Geometry: final body of the model. Coordinates: model frame, mm. Face numbers are marked on the shaded views. A direction names the side the tool comes from. Give positions to 0.01 mm unless a question says otherwise; leave off trailing zeros. Loops run counter-clockwise (first coordinate to the right, second up) from the corner with the lowest first, then second, coordinate; pieces in that order, holes last. Notation, with made-up numbers: (3.5, -23.5) - (16.5, -23.5) arc R27 cw to (16.5, 12.5) - close; hole circle Ø3 at (55, 82.5). An arc over 180 degrees is marked (long way). Use CSV: the item, a comma, the result in double quotes. Start each with the question number.
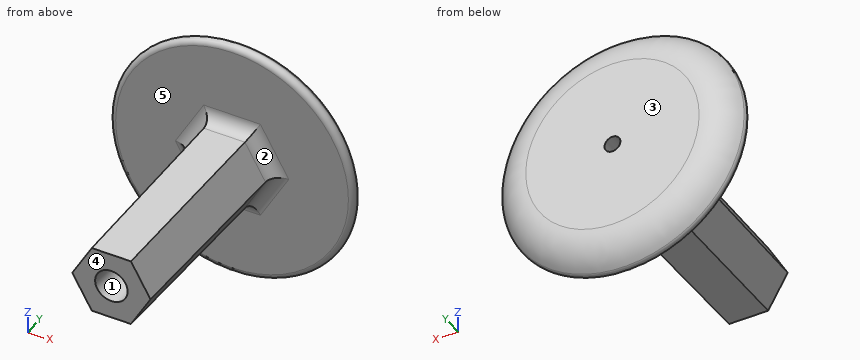
```python
from build123d import *

# Parameters (mm, degrees)
SHAFT_DEPTH          = 22.352
DRAFT_ON_SHAFT_ANGLE = 0.5
SKETCH3_R            = 1.524
THRU_HOLE_DEPTH      = 28.574862156
THRU_HOLE_DRAFT      = -2
FILLET1_R            = 1.27


with BuildPart() as part:
    # Sketch1 → Head (revolve)
    with BuildSketch(Plane.XY, mode=Mode.PRIVATE) as head_sk:
        with BuildLine():
            Line((0, 0), (10.910430592, 0))
            ThreePointArc((10.910430592, 0), (11.355976066, 0.263964694), (11.338496837, 0.781538462))
            ThreePointArc((11.338496837, 0.781538462), (9.958264798, 2.071591054), (8.128, 2.54))
            Line((8.128, 2.54), (0, 2.54))
            Line((0, 2.54), (0, 0))
        make_face()
    revolve(head_sk.sketch.rotate(Axis((0, 2.54, 0), (0, -1, 0)), 180), axis=Axis((0, 2.54, 0), (0, -1, 0)))

    # Sketch2 → Shaft (add)
    with BuildSketch(Plane(origin=(0, 2.54, 0), x_dir=(-1, 0, 0), z_dir=(0, 1, 0))):
        Polygon((1.833087105, -3.175), (-1.833087105, -3.175), (-3.666174209, 0), (-1.833087105, 3.175), (1.833087105, 3.175), (3.666174209, 0), align=None)
    extrude(amount=-SHAFT_DEPTH)

    # Draft on Shaft
    draft_on_shaft_faces = [part.faces().sort_by_distance(p)[0] for p in [
        (0, -9.906, 3.175),
        (2.749630657, -9.906, 1.5875),
        (2.749630657, -9.906, -1.5875),
        (0, -9.906, -3.175),
        (-2.749630657, -9.906, -1.5875),
        (-2.749630657, -9.906, 1.5875),
    ]]
    draft(draft_on_shaft_faces, Plane(origin=(5.499261314, -19.812, 3.175), x_dir=(-1, 0, 0), z_dir=(0, -1, 0)), DRAFT_ON_SHAFT_ANGLE)


with BuildPart() as thru_hole_tool:
    # Sketch3 → Thru Hole (with draft: the straight prism first)
    with BuildSketch(Plane.XZ.offset(19.812)):
        Circle(SKETCH3_R)
    extrude(amount=-THRU_HOLE_DEPTH)
    # Thru Hole: the draft: its side faces are tilted about the plane it starts from
    thru_hole_sides = [thru_hole_tool.faces().sort_by_distance(p)[0] for p in [
        (-1.524, -5.524568922, 0),
    ]]
    draft(thru_hole_sides, Plane.XZ.offset(19.812), THRU_HOLE_DRAFT)


with BuildPart() as part_1:
    add(part.part)

    # Thru Hole: cut by thru_hole_tool
    add(thru_hole_tool.part, mode=Mode.SUBTRACT)

    # Fillet1
    fillet1_edges = [part_1.edges().sort_by_distance(p)[0] for p in [
        (-2.899363595, 0, -1.673948352),
        (0, 0, -3.347896705),
        (2.899363595, 0, 1.673948352),
        (0, 0, 3.347896705),
        (-2.899363595, 0, 1.673948352),
        (2.899363595, 0, -1.673948352),
    ]]
    fillet(fillet1_edges, radius=FILLET1_R)


solid = part_1.part
```
Item 1: Reachability of the marked faces 4 and 5 from +Z, -Z, +X, -X, +Y, -Y: full face, straight path, thin tool, end or side. Return the list, or none.
Item 2: Ray query, probe 1 along Z at (x, y) = (-0.75, -15.75); probe 2 along Y at (x, z) = (-6.75, -3.5); probe 3 along X at (y, z) = (-3, -0.5). Return the intervals inside material, ascending.
Item 3: Section A-A (y = -16). Output: boundary loops of the cut face in (x, z), plus the area to 3 significant figures.
Item 4: Pin query (flat end, axial travel): pin 1 Ø10 at (x, y) = (7, -1.5) entering from -Z; pin 2 Ø6 at (x, y) = (4, -4) entering from -Z; pin 3 Ø3 at (x, y) = (3.5, -7.5) entering from +Z. Return the tip coordinate at first contact, or that it passes through.
Item 5: Section B-B (x = 0). Output: boundary loops of the cut face in (y, z) (1 decimal).
Item 6: Section C-C (y = -2). Output: boundary loops of the cut face in (x, z).
Item 7: Mould query, pull axis X, two halves, no side actions, for the marked faces 1, 2 and 3. Classes: pulls with the +X half, pulls with the -X half, needs draft (parallel to the pull), parting line crosses it, or undercut.
Outcome:
1,face 4,"+Z, -Z, +X, -X, -Y"
1,face 5,"-Y"
2,probe 1,"z = -3.21 to -1.16, 1.16 to 3.21"
2,probe 2,"y = 0 to 2.54"
2,probe 3,"x = -3.55 to -0.79, 0.79 to 3.55"
3,outline,"(-3.7, 0) - (-1.85, -3.21) - (1.85, -3.21) - (3.7, 0) - (1.85, 3.21) - (-1.85, 3.21) - close; hole circle Ø2.78 at (0, 0)"
3,area,"29.6 mm2"
4,pin 1,"stops at z = -11.16"
4,pin 2,"stops at z = -3.33"
4,pin 3,"stops at z = 3.1"
5,outline,"(-19.8, -3.2) - (-1.3, -3.3) arc R1.3 cw to (0, -4.6) - (0, -10.9) arc R0.5 ccw to (0.8, -11.3) arc R3.8 ccw to (2.5, -8.1) - (2.5, -0.7) - (-19.8, -1.5) - close; (-19.8, 1.5) - (2.5, 0.7) - (2.5, 8.1) arc R3.8 ccw to (0.8, 11.3) arc R0.5 ccw to (0, 10.9) - (0, 4.6) arc R1.3 cw to (-1.3, 3.3) - (-19.8, 3.2) - close"
6,outline,"(-3.85, 0) - (-1.92, -3.33) - (1.92, -3.33) - (3.85, 0) - (1.92, 3.33) - (-1.92, 3.33) - close; hole circle Ø1.8 at (0, 0)"
7,face 1,"undercut"
7,face 2,"pulls with the +X half"
7,face 3,"needs draft"
